Can you work these out from the model? Positions are in its coordinate system, mm. Face numbers are marked on the shaded views. A direction names the side the tool comes from. Round coordinates to 2 decimals unless told otherwise and drop trailing zeros. Loops run counter-clockwise (first coordinate to the right, second up) from the corner with the lowest first, then second, coordinate; pieces in that order, holes last.
from build123d import *

# Parameters (mm, degrees)
M3X0_5_TAPPED_HOLE1_D     = 2.5
M3X0_5_TAPPED_HOLE1_DEPTH = 7.5
M3X0_5_TAPPED_HOLE1_TIP   = 0.751075774
CUT_EXTRUDE1_START        = -14
CUT_EXTRUDE1_DEPTH        = 14


with BuildPart() as part:
    # Sketch1 → Revolve1 (revolve)
    with BuildSketch(Plane.XY, mode=Mode.PRIVATE) as revolve1_sk:
        Polygon((0, 0), (0, 3), (14, 3), (14, 6), (17.9, 6), (17.9, 11), (99.4, 11), (99.4, 0), align=None)
    revolve(revolve1_sk.sketch.rotate(Axis((0, 0, 0), (1, 0, 0)), 90), axis=Axis((0, 0, 0), (1, 0, 0)))

    # M3x0.5 Tapped Hole1
    with Locations(Plane.ZY.offset(-17.9)):
        with Locations((-9, 0), (0, 9), (9, 0), (0, -9)):
            Hole(M3X0_5_TAPPED_HOLE1_D / 2, depth=M3X0_5_TAPPED_HOLE1_DEPTH)
            with Locations((0, 0, -(M3X0_5_TAPPED_HOLE1_DEPTH + M3X0_5_TAPPED_HOLE1_TIP / 2))):  # 118° drill point
                Cone(0, M3X0_5_TAPPED_HOLE1_D / 2, M3X0_5_TAPPED_HOLE1_TIP, mode=Mode.SUBTRACT)

    # Sketch4 → Cut-Extrude1 (cut)
    with BuildSketch(Plane.ZY.offset(CUT_EXTRUDE1_START)):
        with BuildLine():
            Line((-1.658312395, 2.5), (1.658312395, 2.5))
            ThreePointArc((1.658312395, 2.5), (0, 3), (-1.658312395, 2.5))
        make_face()
    extrude(amount=CUT_EXTRUDE1_DEPTH, mode=Mode.SUBTRACT)


solid = part.part
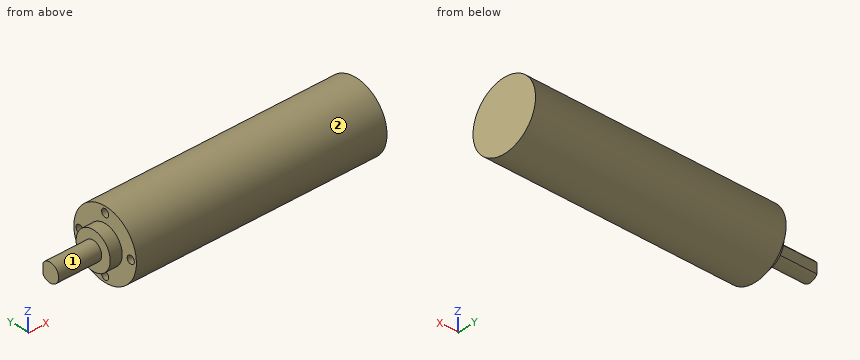
(1) Will these pins go through, and if not, where does the flat tip stop? P1, Ø3, axis at x = 56.5, z = 0.5, coming from the -Y side; P2, Ø1.5, axis at x = 76.5, y = 5, coming from the -Z side; P3, Ø4, axis at y = 2, z = -6.5, coming from the -X side; P4, Ø3, axis at x = 17.5, y = 3, coming from the -Z side.
Worked answers:
P1: stops at y = -11
P2: stops at z = -10.15
P3: stops at x = 14
P4: stops at z = -10.89
(2) If I drill on line 1 (Y direction, x = 22, z = 0); line 2 (Y direction, x = 49, z = 0); line 3 (X direction, y = -6, z = 1), over which ranges is the centre line in solid material (lowest first)?
Worked answers:
line 1: y = -11 to -10.25, -7.75 to 7.75, 10.25 to 11
line 2: y = -11 to 11
line 3: x = 17.9 to 99.4
(3) If we section it at A-A, the plane x = 22: List the corners of the cut face in (y, z) for me, then the cut area to 3 significant figures.
Worked answers:
outline: circle Ø22 at (0, 0); hole circle Ø2.5 at (-9, 0); hole circle Ø2.5 at (0, -9); hole circle Ø2.5 at (0, 9); hole circle Ø2.5 at (9, 0)
area: 360 mm2
(4) If we section it at C-C, the plane x = 77: List the corners of the cut face in (y, z) for me.
Worked answers:
outline: circle Ø22 at (0, 0)
(5) If we section it at B-B, the plane x = 6: List the corners of the cut face in (y, z) for me.
Worked answers:
outline: (2.5, -1.66) - (2.5, 1.66) arc R3 ccw (long way) to start
(6) For the marked faces 1 and 2, which set-ups out of +Z, -Z, +X, -X, +Y, -Y let a thin tool reach every point of the face, with its end or its side?
Worked answers:
face 1: -X
face 2: +X, -X
